Geometry: final body of the model. Coordinates: model frame, mm. A direction names the side the tool comes from. Round coordinates to 2 decimals unless told otherwise and drop trailing zeros. Write each loop counter-clockwise with the first axis right and the second up, starting at its lowest first coordinate (ties: lowest second). Pieces come first, ordered by that corner, then holes. Notation, with made-up numbers: (-9.5, 45) -> (9.5, 45) arc R33 cw to (9.5, 80) -> close; hole circle Ø10 at (72, -2.5). An arc over 180 degrees is marked (long way). One line per item, written item: value. Start each with the question number.
from build123d import *

# Parameters (mm, degrees)
SKETCH_1_W      = 40
SKETCH_1_H      = 16
EXTRUDE_1_DEPTH = 100
SKETCH_2_W      = 40
SKETCH_2_H      = 30
EXTRUDE_2_DEPTH = 200
SKETCH_3_W      = 40
SKETCH_3_H      = 35
EXTRUDE_3_DEPTH = 200


with BuildPart() as part:
    # 草图1 → 凸台-拉伸1 (new body)
    with BuildSketch(Plane(origin=(0, 0, 0), x_dir=(1, 0, 0), z_dir=(0, 1, 0))):
        Rectangle(SKETCH_1_W, SKETCH_1_H)
    extrude(amount=EXTRUDE_1_DEPTH)

    # 草图2 → 凸台-拉伸2 (add)
    with BuildSketch(Plane.XY.offset(8)):
        with Locations((0, 15)):
            Rectangle(SKETCH_2_W, SKETCH_2_H)
    extrude(amount=EXTRUDE_2_DEPTH)

    # 草图3 → 凸台-拉伸3 (add)
    with BuildSketch(Plane(origin=(0, 30, 0), x_dir=(1, 0, 0), z_dir=(0, 1, 0))):
        with Locations((0, -190.5)):
            Rectangle(SKETCH_3_W, SKETCH_3_H)
    extrude(amount=EXTRUDE_3_DEPTH)


solid = part.part
(1) Section query B-B (y = 189). Output: boundary loops of the cut face in (x, z), and give its area (3 significant figures).
(2) Pin query (flat end, axial travel): pin 1 (2 mm diameter, centred on x = 3, z = 118.5, fed in from +Y); pin 2 (17.5 mm diameter, centred on x = 5, z = 4, fed in from +Y); pin 3 (8 mm diameter, centred on x = -14.5, z = 86, fed in from -Y); pin 4 (12 mm diameter, centred on x = -1.5, y = 116.5, fed in from -Z). Return the tip coordinate at first contact, or that it passes through.
(3) Pull-direction query (Z, two-part tool) for faces 1 (the face through (0, 65, 8)), 2 (the face through (0, 113, 208)), 3 (the face through (0, 0, 98)); classes: pulls with the +Z half, pulls with the -Z half, needs draft (parallel to the pull), parting line crosses it, or undercut.
(4) Section query A-A (x = -14). Output: boundary loops of the cut face in (y, z).
(5) Section query C-C (z = 164). Output: boundary loops of the cut face in (x, y), and give its area (3 significant figures).
(6) Line query: probe 1 along Z at (x, y) = (7, 35.5); probe 2 along Z at (x, y) = (18, 135); probe 3 along Y at (x, z) = (18, 38). Output: solid intervals per line, ascending.
(7) Set-up query: faces 4 (the face through (0, 230, 190)), 5 (the face through (0, 129, 173)), 6 (the face through (0, 100, 0)). Return all of +Z, -Z, +X, -X, +Y, -Y with unobstructed straight access to the full face (end or side cutting, diameter ignored); none if empty.
Results list:
1. outline: (-20, 173) -> (20, 173) -> (20, 208) -> (-20, 208) -> close
1. area: 1,400 mm^2
2. pin 1: stops at y = 30
2. pin 2: stops at y = 100
2. pin 3: stops at y = 0
2. pin 4: stops at z = 173
3. face 1: undercut
3. face 2: pulls with the +Z half
3. face 3: needs draft
4. outline: (0, -8) -> (100, -8) -> (100, 8) -> (30, 8) -> (30, 173) -> (230, 173) -> (230, 208) -> (0, 208) -> close
5. outline: (-20, 0) -> (20, 0) -> (20, 30) -> (-20, 30) -> close
5. area: 1,200 mm^2
6. probe 1: z = -8 to 8, 173 to 208
6. probe 2: z = 173 to 208
6. probe 3: y = 0 to 30
7. face 4: +Z, -Z, +X, -X, +Y
7. face 5: +X, -X, +Y
7. face 6: -Z, +X, -X, +Y
